from build123d import *

# Parameters (mm, degrees)
BOSS_EXTRUDE1_DEPTH    = 4
SKETCH3_W              = 76
SKETCH3_H              = 4
BOSS_EXTRUDE2_DEPTH    = 56.4
SKETCH15_R             = 2.5
SKETCH15_R_2           = 19.5
CUT_EXTRUDE3_DEPTH     = 88.224308538
FILLET4_R              = 4
SKETCH18_R             = 1.5
CUT_EXTRUDE4_DEPTH     = 96.708933752
CONVERT_SOLID2_START   = -28.2
CONVERT_SOLID2_DEPTH   = 56.4
CONVERT_SOLID2_2_DEPTH = 56.4


# Read off the part's stored shape, not the designer's step: Convert-Solid2
with BuildPart() as part:
    # Sketch1 → Boss-Extrude1 (new body)
    with BuildSketch(Plane.XY):
        with BuildLine():
            Line((28.2, -28.2), (-28.2, -28.2))
            Line((-28.2, -28.2), (-28.2, 24.2))
            ThreePointArc((-28.2, 24.2), (-27.028427125, 27.028427125), (-24.2, 28.2))
            Line((-24.2, 28.2), (24.2, 28.2))
            ThreePointArc((24.2, 28.2), (27.028427125, 27.028427125), (28.2, 24.2))
            Line((28.2, 24.2), (28.2, -28.2))
        make_face()
    extrude(amount=BOSS_EXTRUDE1_DEPTH)

    # Sketch3 → Boss-Extrude2 (add)
    with BuildSketch(Plane(origin=(28.2, 0, 0), x_dir=(0, 0, -1), z_dir=(1, 0, 0))):
        with Locations((34, -30.2)):
            Rectangle(SKETCH3_W, SKETCH3_H)
    extrude(amount=-BOSS_EXTRUDE2_DEPTH)

    # Sketch15 → Cut-Extrude3 (cut, through all)
    with BuildSketch(Plane.XY.offset(4)):
        with Locations((-23.57, 23.57)):
            Circle(SKETCH15_R)
        with Locations((23.57, 23.57)):
            Circle(SKETCH15_R)
        Circle(SKETCH15_R_2)
    extrude(amount=-CUT_EXTRUDE3_DEPTH, mode=Mode.SUBTRACT)

    # Fillet4
    fillet4_edges = [part.edges().sort_by_distance(p)[0] for p in [
        (-28.2, -30.2, -72),
        (28.2, -30.2, -72),
    ]]
    fillet(fillet4_edges, radius=FILLET4_R)

    # Sketch18 → Cut-Extrude4 (cut, through all)
    with BuildSketch(Plane(origin=(0, -28.2, 0), x_dir=(1, 0, 0), z_dir=(0, 1, 0))):
        with Locations(Location((-24.2, 68, 0), (0, 0, 270))):
            Circle(SKETCH18_R)
        with Locations(Location((24.2, 68, 0), (0, 0, 270))):
            Circle(SKETCH18_R)
        with Locations(Location((-24.2, 23, 0), (0, 0, 270))):
            Circle(SKETCH18_R)
        with Locations(Location((24.2, 23, 0), (0, 0, 270))):
            Circle(SKETCH18_R)
    extrude(amount=-CUT_EXTRUDE4_DEPTH, mode=Mode.SUBTRACT)

    # Convert-Solid2 outline → Convert-Solid2 (cut)
    with BuildSketch(Plane.YZ.offset(CONVERT_SOLID2_START)):
        with BuildLine():
            ThreePointArc((-32.2, -4), (-29.856854249, 1.656854249), (-24.2, 4))
            Line((-24.2, 4), (-32.2, 4))
            Line((-32.2, 4), (-32.2, -4))
        make_face()
    extrude(amount=CONVERT_SOLID2_DEPTH, mode=Mode.SUBTRACT)

    # Convert-Solid2 2 outline → Convert-Solid2 2 (add)
    with BuildSketch(Plane.YZ.offset(CONVERT_SOLID2_START)):
        with BuildLine():
            ThreePointArc((-28.2, -4), (-27.028427125, -1.171572875), (-24.2, 0))
            Line((-24.2, 0), (-28.2, 0))
            Line((-28.2, 0), (-28.2, -4))
        make_face()
    extrude(amount=CONVERT_SOLID2_2_DEPTH)


solid = part.part
Work out the finished part from the listing and answer in its coordinate system (mm). A direction names the side the tool comes from. Give positions to 0.01 mm unless a question says otherwise; leave off trailing zeros. Order: outer loops, then holes, each group sorted by start corner. A loop starts at its lowest first (then second) coordinate and runs counter-clockwise, first axis right, second up. Notation, with made-up numbers: (61.25, 4.25) -> (113.25, 4.25) arc R25 cw to (113.25, 33.25) -> close; hole circle Ø7 at (-4, 39.25). An arc over 180 degrees is marked (long way). One line per item, written item: value.
Item 1: Find section D-D, the plane y = -9. Give the vertices of the cut face in (x, z).
Answer sheet:
outline: (-28.2, 0) -> (-17.3, 0) -> (-17.3, 4) -> (-28.2, 4) -> close; (17.3, 0) -> (28.2, 0) -> (28.2, 4) -> (17.3, 4) -> close
Item 2: A tool of negligible diameter and unlimited length cuts with its end or side. For faces 1 (the cylindrical face through (24.65, -30.17, -66.57)), 2 (the flat face through (0, -28.2, -38)), from which of +Z, -Z, +X, -X, +Y, -Y can it reach the whole face along a straight path? Write none if from no direction.
Answer sheet:
face 1: +Y, -Y
face 2: -Z, +X, -X, +Y
Item 3: Find section B-B, the plane y = 7. Give the vertices of the cut face in (x, z), plus the area to 3 significant figures.
Answer sheet:
outline: (-28.2, 0) -> (-18.2, 0) -> (-18.2, 4) -> (-28.2, 4) -> close; (18.2, 0) -> (28.2, 0) -> (28.2, 4) -> (18.2, 4) -> close
area: 80.0 mm²
Item 4: Flat-ended cylindrical pins translate along their axes: P1, Ø6.5, axis at x = 23.57, y = 23.57, coming from the -Z side; P2, Ø5, axis at x = -24.2, z = -23, coming from the +Y side. Find the tip coordinate at first contact, or state that the pin passes through.
Answer sheet:
P1: z = 0
P2: y = -28.2
Item 5: Find section C-C, the plane z = -45.5. Give the vertices of the cut face in (x, y), plus the area to 3 significant figures.
Answer sheet:
outline: (-28.2, -32.2) -> (28.2, -32.2) -> (28.2, -28.2) -> (-28.2, -28.2) -> close
area: 226 mm²
Item 6: Straight lines are drawn through the part: probe 1 along X at (y, z) = (-31, -23); probe 2 along Y at (x, z) = (10.5, -10); probe 3 along Y at (x, z) = (0, 3.05). For each, find the intervals that lie inside material, in ascending order.
Answer sheet:
probe 1: -28.2 to -25.7, -22.7 to 22.7, 25.7 to 28.2
probe 2: -32.2 to -28.2
probe 3: -27.98 to -19.5, 19.5 to 28.2
Item 7: Determine the mould class of faces 3 (the cylindrical face through (-25.664, -30.172, -23.325)), 4 (the cylindrical face through (-27.059, -30.172, -70.797)), 5 (the flat face through (-28.2, -29, -16)), 6 (the cylindrical face through (25.21, -30.17, -24.11)) for opening direction Z: released by +Z, released by -Z, zero draft, split by the parting line, or undercut.
Answer sheet:
face 3: undercut
face 4: released by -Z
face 5: zero draft
face 6: undercut
Item 8: Find section A-A, the plane x = 7.5. Give the vertices of the cut face in (y, z).
Answer sheet:
outline: (-32.2, -72) -> (-28.2, -72) -> (-28.2, -4) arc R4 cw to (-24.2, 0) -> (-18, 0) -> (-18, 4) -> (-24.2, 4) arc R8 ccw to (-32.2, -4) -> close; (18, 0) -> (28.2, 0) -> (28.2, 4) -> (18, 4) -> close
